Source: CAD feature listing. Evaluate the final solid. Frame: model axes, mm. Face numbers are marked on the shaded views. A direction names the side the tool comes from. Round coordinates to 2 decimals unless told otherwise and drop trailing zeros. Write each loop counter-clockwise with the first axis right and the second up, starting at its lowest first coordinate (ties: lowest second). Pieces come first, ordered by that corner, then holes. Notation, with made-up numbers: M 77,-15.5 L 88,-15.5 A27 ccw 88,4.5 Z; hole C -15.5,-28.5 d1. An arc over 180 degrees is marked long. Use a Markdown table: item, result.
```python
from build123d import *

# Parameters (mm, degrees)
EXTRUDE_1_DEPTH     = 5
SKETCH_2_R          = 6.5
EXTRUDE_2_DEPTH     = 15
SKETCH_5_OUTSIDE_W  = 29.584
SKETCH_5_OUTSIDE_H  = 26.8
SKETCH_5_OUTSIDE_R  = 10
CUT_EXTRUDE_1_DEPTH = 21.346989949
CHAMFER_1_SIZE      = 1
M10X1_25_1_D        = 8.8


with BuildPart() as part:
    # 草图1 → 凸台-拉伸1 (new body)
    with BuildSketch(Plane.XY):
        Polygon((10.392304845, 0), (5.196152423, 9), (-5.196152423, 9), (-10.392304845, 0), (-5.196152423, -9), (5.196152423, -9), align=None)
    extrude(amount=EXTRUDE_1_DEPTH)

    # 草图2 → 凸台-拉伸2 (add)
    with BuildSketch(Plane.XY.offset(5)):
        Circle(SKETCH_2_R)
    extrude(amount=EXTRUDE_2_DEPTH)

    # 草图5 outside → 切除-拉伸1 (cut, through all)
    with BuildSketch(Plane.XY.offset(5)):
        Rectangle(SKETCH_5_OUTSIDE_W, SKETCH_5_OUTSIDE_H)
        Circle(SKETCH_5_OUTSIDE_R, mode=Mode.SUBTRACT)
    extrude(amount=-CUT_EXTRUDE_1_DEPTH, mode=Mode.SUBTRACT)

    # 倒角1
    chamfer_1_edges = [part.edges().sort_by_distance(p)[0] for p in [
        (-6.5, 0, 20),
    ]]
    chamfer(chamfer_1_edges, length=CHAMFER_1_SIZE)

    # M10x1.25 螺纹孔1 (through all)
    with Locations(Plane.XY.offset(20)):
        with Locations((0, 0)):
            Hole(M10X1_25_1_D / 2)


solid = part.part
```
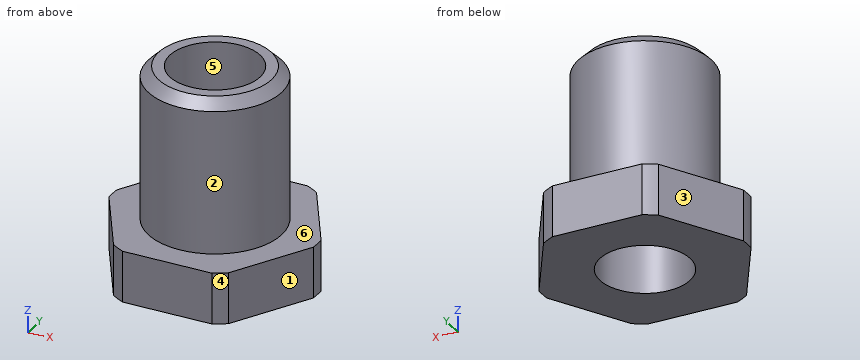
Q1. Line query: L1, parallel to Y at x = -0.25, z = 12.5; L2, parallel to Z at x = 0, y = -7.5; L3, parallel to X at y = -1.75, z = 18.25. Output: solid intervals per line, ascending.
Results are:
| item | result |
|---|---|
| L1 | -6.5 to -4.39, 4.39 to 6.5 |
| L2 | 0 to 5 |
| L3 | -6.26 to -4.04, 4.04 to 6.26 |
Q2. Section D-D on x = 7.25. Return loops of the section in (y, z).
Results are:
| item | result |
|---|---|
| outline | M -5.44,0 L 5.44,0 L 5.44,5 L -5.44,5 Z |
Q3. Section B-B on x = 0. Return loops of the section in (y, z), plus the area to 3 significant figures.
Results are:
| item | result |
|---|---|
| outline | M -9,0 L -4.4,0 L -4.4,20 L -5.5,20 L -6.5,19 L -6.5,5 L -9,5 Z; M 4.4,0 L 9,0 L 9,5 L 6.5,5 L 6.5,19 L 5.5,20 L 4.4,20 Z |
| area | 108 mm^2 |
Q4. First-contact query: pin 1 Ø6 at (x, y) = (4, 1.5) entering from -Z; pin 2 Ø6 at (y, z) = (-4.5, 17) entering from -X; pin 3 Ø1.5 at (x, z) = (-2, 7.5) entering from -Y; pin 4 Ø6 at (y, z) = (-3, 8.5) entering from -X. Flat tips, straight axial feed; report the tip coordinate or a pass-through.
Results are:
| item | result |
|---|---|
| pin 1 | z = 0 |
| pin 2 | x = -6.32 |
| pin 3 | y = -6.38 |
| pin 4 | x = -6.5 |
Q5. Reachability of the marked faces 1 and 2 from +Z, -Z, +X, -X, +Y, -Y: full face, straight path, thin tool, end or side. Return the list, or none.
Results are:
| item | result |
|---|---|
| face 1 | +Z, -Z, +X, -Y |
| face 2 | +Z |
Q6. Section A-A on y = 0. Return loops of the section in (x, z).
Results are:
| item | result |
|---|---|
| outline | M -10,0 L -4.4,0 L -4.4,20 L -5.5,20 L -6.5,19 L -6.5,5 L -10,5 Z; M 4.4,0 L 10,0 L 10,5 L 6.5,5 L 6.5,19 L 5.5,20 L 4.4,20 Z |
Q7. Mould query, pull axis X, two halves, no side actions, for the marked faces 3, 4, 5 and 6. Classes: +X half, -X half, draft (parallel to the pull), parting line (faces both ways), or undercut.
Results are:
| item | result |
|---|---|
| face 3 | -X half |
| face 4 | +X half |
| face 5 | undercut |
| face 6 | draft |
Q8. Section C-C on z = 3.5. Return loops of the section in (x, y).
Results are:
| item | result |
|---|---|
| outline | M -9.97,-0.73 L -5.61,-8.27 A10 ccw -4.36,-9 L 4.36,-9 A10 ccw 5.61,-8.27 L 9.97,-0.73 A10 ccw 9.97,0.73 L 5.61,8.27 A10 ccw 4.36,9 L -4.36,9 A10 ccw -5.61,8.27 L -9.97,0.73 A10 ccw Z; hole C 0,0 d8.8 |
